from build123d import *

# Parameters (mm, degrees)
SKETCH1_W                                        = 187.5
SKETCH1_H                                        = 12.5
BOSS_EXTRUDE1_DEPTH                              = 25
CBORE_FOR_1_4_SOCKET_HEAD_CAP_SCREW1_D           = 6.7564
CBORE_FOR_1_4_SOCKET_HEAD_CAP_SCREW1_CBORE_D     = 11.1125
CBORE_FOR_1_4_SOCKET_HEAD_CAP_SCREW1_CBORE_DEPTH = 6.35
CUT_EXTRUDE1_REACH                               = 176.672
SKETCH4_R                                        = 4.445
SKETCH4_R_2                                      = 6.35
F_1_4_20_TAPPED_HOLE1_D                          = 5.1054


with BuildPart() as part:
    # Sketch1 → Boss-Extrude1 (new body)
    with BuildSketch(Plane(origin=(0, 0, 0), x_dir=(1, 0, 0), z_dir=(0, 1, 0))):
        with Locations((78.671443618, -0.761090319)):
            Rectangle(SKETCH1_W, SKETCH1_H)
    extrude(amount=BOSS_EXTRUDE1_DEPTH)

    # CBORE for 1/4 Socket Head Cap Screw1 (through all)
    with Locations(Plane(origin=(9.921443618, 25, 0.761090319), x_dir=(0, 0, 1), z_dir=(0, 1, 0))):
        with Locations((0, 0), (0, 150.000000108)):
            CounterBoreHole(CBORE_FOR_1_4_SOCKET_HEAD_CAP_SCREW1_D / 2, CBORE_FOR_1_4_SOCKET_HEAD_CAP_SCREW1_CBORE_D / 2, CBORE_FOR_1_4_SOCKET_HEAD_CAP_SCREW1_CBORE_DEPTH)

    # Sketch4 → Cut-Extrude1 (cut, up to next)
    with BuildSketch(Plane(origin=(0, 0, -5.488909681), x_dir=(-1, 0, 0), z_dir=(0, 0, -1)), mode=Mode.PRIVATE) as cut_extrude1_sk1:
        with BuildLine():
            ThreePointArc((-30.476443618, 16.11), (-34.921443618, 20.555), (-39.366443618, 16.11))
            Line((-39.366443618, 16.11), (-30.476443618, 16.11))
        make_face()
    cut_extrude1_tool1 = extrude(cut_extrude1_sk1.sketch, amount=-CUT_EXTRUDE1_REACH, mode=Mode.PRIVATE) & part.part
    # Sketch4 → Cut-Extrude1 (cut, up to next)
    with BuildSketch(Plane(origin=(0, 0, -5.488909681), x_dir=(-1, 0, 0), z_dir=(0, 0, -1)), mode=Mode.PRIVATE) as cut_extrude1_sk2:
        with BuildLine():
            Line((-30.476443618, 16.11), (-39.366443618, 16.11))
            ThreePointArc((-39.366443618, 16.11), (-34.921443618, 11.665), (-30.476443618, 16.11))
        make_face()
    cut_extrude1_tool2 = extrude(cut_extrude1_sk2.sketch, amount=-CUT_EXTRUDE1_REACH, mode=Mode.PRIVATE) & part.part
    # Sketch4 → Cut-Extrude1 (cut, up to next)
    with BuildSketch(Plane(origin=(0, 0, -5.488909681), x_dir=(-1, 0, 0), z_dir=(0, 0, -1)), mode=Mode.PRIVATE) as cut_extrude1_sk3:
        with BuildLine():
            ThreePointArc((-30.476443618, 16.11), (-34.921443618, 20.555), (-39.366443618, 16.11))
            Line((-39.366443618, 16.11), (-30.476443618, 16.11))
        make_face()
    cut_extrude1_tool3 = extrude(cut_extrude1_sk3.sketch, amount=-CUT_EXTRUDE1_REACH, mode=Mode.PRIVATE) & part.part
    # Sketch4 → Cut-Extrude1 (cut, up to next)
    with BuildSketch(Plane(origin=(0, 0, -5.488909681), x_dir=(-1, 0, 0), z_dir=(0, 0, -1)), mode=Mode.PRIVATE) as cut_extrude1_sk4:
        with BuildLine():
            Line((-30.476443618, 16.11), (-39.366443618, 16.11))
            ThreePointArc((-39.366443618, 16.11), (-34.921443618, 11.665), (-30.476443618, 16.11))
        make_face()
    cut_extrude1_tool4 = extrude(cut_extrude1_sk4.sketch, amount=-CUT_EXTRUDE1_REACH, mode=Mode.PRIVATE) & part.part
    # Sketch4 → Cut-Extrude1 (cut, up to next)
    with BuildSketch(Plane(origin=(0, 0, -5.488909681), x_dir=(-1, 0, 0), z_dir=(0, 0, -1)), mode=Mode.PRIVATE) as cut_extrude1_sk5:
        with Locations((-122.421443618, 16.11)):
            Circle(SKETCH4_R)
    cut_extrude1_tool5 = extrude(cut_extrude1_sk5.sketch, amount=-CUT_EXTRUDE1_REACH, mode=Mode.PRIVATE) & part.part
    # Sketch4 → Cut-Extrude1 (cut, up to next)
    with BuildSketch(Plane(origin=(0, 0, -5.488909681), x_dir=(-1, 0, 0), z_dir=(0, 0, -1)), mode=Mode.PRIVATE) as cut_extrude1_sk6:
        with Locations((-78.671443618, 16.11)):
            Circle(SKETCH4_R_2)
    cut_extrude1_tool6 = extrude(cut_extrude1_sk6.sketch, amount=-CUT_EXTRUDE1_REACH, mode=Mode.PRIVATE) & part.part
    add(cut_extrude1_tool1.solids().sort_by_distance((34.921444, 17.996517, -5.48891))[0], mode=Mode.SUBTRACT)
    add(cut_extrude1_tool2.solids().sort_by_distance((34.921444, 14.223483, -5.48891))[0], mode=Mode.SUBTRACT)
    add(cut_extrude1_tool3.solids().sort_by_distance((34.921444, 17.996517, -5.48891))[0], mode=Mode.SUBTRACT)
    add(cut_extrude1_tool4.solids().sort_by_distance((34.921444, 14.223483, -5.48891))[0], mode=Mode.SUBTRACT)
    add(cut_extrude1_tool5.solids().sort_by_distance((122.421444, 16.11, -5.48891))[0], mode=Mode.SUBTRACT)
    add(cut_extrude1_tool6.solids().sort_by_distance((78.671444, 16.11, -5.48891))[0], mode=Mode.SUBTRACT)

    # 1/4-20 Tapped Hole1 (through all)
    with Locations(Plane(origin=(78.671443618, 25, 0.761090319), x_dir=(0, 0, 1), z_dir=(0, 1, 0))):
        with Locations((0, 0)):
            Hole(F_1_4_20_TAPPED_HOLE1_D / 2)


solid = part.part
Build history of the part. All positions in model axes, mm. A direction names the side the tool comes from. Give positions to 0.01 mm unless a question says otherwise; leave off trailing zeros. Write each loop counter-clockwise with the first axis right and the second up, starting at its lowest first coordinate (ties: lowest second). Pieces come first, ordered by that corner, then holes. Notation, with made-up numbers: (74, -20) - (104, -20) arc R23 cw to (104, -12) - close; hole circle Ø9 at (55.5, 69). An arc over 180 degrees is marked (long way). Use one line per item in the form item = value. Start each with the question number.
1. 3-axis set-ups, long thin cutter, end or side, ignore diameter. For faces 4 (the face through (4.497, 21.869, -0.443)), 5 (the face through (39.03, 17.81, 0.67)): which of +Z, -Z, +X, -X, +Y, -Y reach the whole face in a straight line?
2. Probe line 1 (X direction, y = 2.75, z = 0.75); line 2 (X direction, y = 4.5, z = 1.75); line 3 (X direction, y = 24.25, z = -2.5). List the from-to ranges inside material, lowest first. Write a range as [from, to].
3. Two-plate mould, pull along Z, no slides. Class faces 1 (the face through (77.4, 9.5, 7.011)), 2 (the face through (-15.079, 12, 1)), 3 (the face through (13.27, 9.19, 1.2)): released by +Z, released by -Z, zero draft, split by the parting line, or undercut.
4. Band-saw the part on C-C on y = 6.75. Write the cut outline in (x, z), plus the area to 3 significant figures.
5. Band-saw the part on B-B on z = 0.25. Count the separate pieces of the cut face and the enclosed holes in it, plus the area to 3 significant figures.
6. Band-saw the part on A-A on y = 16.11. Write the cut outline in (x, z).
Conclusion:
q1.face_4 = +Y
q1.face_5 = +Z, -Z
q2.line_1 = [-15.08, 6.54], [13.3, 76.12], [81.22, 156.54], [163.3, 172.42]
q2.line_2 = [-15.08, 6.69], [13.15, 76.32], [81.02, 156.69], [163.15, 172.42]
q2.line_3 = [-15.08, 5.42], [14.42, 155.42], [164.42, 172.42]
q3.face_1 = released by +Z
q3.face_2 = zero draft
q3.face_3 = undercut
q4.outline = (-15.08, -5.49) - (172.42, -5.49) - (172.42, 7.01) - (-15.08, 7.01) - close; hole circle Ø6.76 at (9.92, 0.76); hole circle Ø5.11 at (78.67, 0.76); hole circle Ø6.76 at (159.92, 0.76)
q4.area = 2,250 mm²
q5.separate_pieces = 4
q5.enclosed_holes = 2
q5.area = 3,980 mm²
q6.outline = (-15.08, -5.49) - (30.48, -5.49) - (30.48, 7.01) - (-15.08, 7.01) - close; (39.37, -5.49) - (72.32, -5.49) - (72.32, 7.01) - (39.37, 7.01) - close; (85.02, -5.49) - (117.98, -5.49) - (117.98, 7.01) - (85.02, 7.01) - close; (126.87, -5.49) - (172.42, -5.49) - (172.42, 7.01) - (126.87, 7.01) - close; hole circle Ø6.76 at (9.92, 0.76); hole circle Ø6.76 at (159.92, 0.76)
